Here's how the part is built. I have some questions about the finished solid (model axes, mm). A direction names the side the tool comes from. Give positions to 0.01 mm unless a question says otherwise; leave off trailing zeros. Write each loop counter-clockwise with the first axis right and the second up, starting at its lowest first coordinate (ties: lowest second). Pieces come first, ordered by that corner, then holes. Notation, with made-up numbers: M -28,84 L 22,84 A19 cw 22,106 Z; hole C 47,28.25 d1. An arc over 180 degrees is marked long. Use one line per item in the form item = value. Start each with the question number.
from build123d import *

# Parameters (mm, degrees)
F1_DEPTH = 130
F0_R     = 15
F2_DEPTH = 10
F0_R_2   = 10
F0_R_3   = 5
F3_DEPTH = 5
F4_R     = 0.8
F5_R     = 5


with BuildPart() as f1:
    # F0 (on Top) → F1 (new body)
    with BuildSketch(Plane.XY):
        with BuildLine():
            ThreePointArc((-137.9369372874, 168.1235290214), (-141.4724711934, 166.6590629273), (-142.9369372874, 163.1235290214))
            Line((-142.9369372874, 163.1235290214), (-142.9369372874, -66.8764709786))
            ThreePointArc((-142.9369372874, -66.8764709786), (-141.4724711934, -70.4120048845), (-137.9369372874, -71.8764709786))
            Line((-137.9369372874, -71.8764709786), (152.0630627126, -71.8764709786))
            ThreePointArc((152.0630627126, -71.8764709786), (155.5985966185, -70.4120048845), (157.0630627126, -66.8764709786))
            Line((157.0630627126, -66.8764709786), (157.0630627126, 163.1235290214))
            ThreePointArc((157.0630627126, 163.1235290214), (155.5985966185, 166.6590629273), (152.0630627126, 168.1235290214))
            Line((152.0630627126, 168.1235290214), (-137.9369372874, 168.1235290214))
        make_face()
        with BuildLine():
            ThreePointArc((-137.9369372874, 153.1235290214), (-135.0080050993, 160.1945968333), (-127.9369372874, 163.1235290214))
            Line((-127.9369372874, 163.1235290214), (92.0630627126, 163.1235290214))
            Line((92.0630627126, 163.1235290214), (142.0630627126, 163.1235290214))
            ThreePointArc((142.0630627126, 163.1235290214), (149.1341305244, 160.1945968333), (152.0630627126, 153.1235290214))
            Line((152.0630627126, 153.1235290214), (152.0630627126, -56.8764709786))
            ThreePointArc((152.0630627126, -56.8764709786), (149.1341305244, -63.9475387905), (142.0630627126, -66.8764709786))
            Line((142.0630627126, -66.8764709786), (92.0630627126, -66.8764709786))
            Line((92.0630627126, -66.8764709786), (-127.9369372874, -66.8764709786))
            ThreePointArc((-127.9369372874, -66.8764709786), (-135.0080050993, -63.9475387905), (-137.9369372874, -56.8764709786))
            Line((-137.9369372874, -56.8764709786), (-137.9369372874, 153.1235290214))
        make_face(mode=Mode.SUBTRACT)
    extrude(amount=F1_DEPTH)

    # F0 (on Top) → F2 (join)
    with BuildSketch(Plane.XY):
        with BuildLine():
            Line((92.0630627126, 163.1235290214), (-127.9369372874, 163.1235290214))
            ThreePointArc((-127.9369372874, 163.1235290214), (-135.0080050993, 160.1945968333), (-137.9369372874, 153.1235290214))
            Line((-137.9369372874, 153.1235290214), (-137.9369372874, -56.8764709786))
            ThreePointArc((-137.9369372874, -56.8764709786), (-135.0080050993, -63.9475387905), (-127.9369372874, -66.8764709786))
            Line((-127.9369372874, -66.8764709786), (92.0630627126, -66.8764709786))
            Line((92.0630627126, -66.8764709786), (92.0630627126, 163.1235290214))
        make_face()
        with Locations((-22.9369372874, 48.1235290214)):
            Circle(F0_R, mode=Mode.SUBTRACT)
        with BuildLine():
            Line((142.0630627126, 163.1235290214), (92.0630627126, 163.1235290214))
            Line((92.0630627126, 163.1235290214), (92.0630627126, -66.8764709786))
            Line((92.0630627126, -66.8764709786), (142.0630627126, -66.8764709786))
            ThreePointArc((142.0630627126, -66.8764709786), (149.1341305244, -63.9475387905), (152.0630627126, -56.8764709786))
            Line((152.0630627126, -56.8764709786), (152.0630627126, 153.1235290214))
            ThreePointArc((152.0630627126, 153.1235290214), (149.1341305244, 160.1945968333), (142.0630627126, 163.1235290214))
        make_face()
    extrude(amount=F2_DEPTH)



with BuildPart() as f2:
    # F0 (on Top) → F2, piece 2 (new body)
    with BuildSketch(Plane.XY):
        with Locations((-22.9369372874, 48.1235290214)):
            Circle(F0_R_2)
        with Locations((-22.9369372874, 48.1235290214)):
            Circle(F0_R_3, mode=Mode.SUBTRACT)
    extrude(amount=F2_DEPTH)


with BuildPart() as f1_1:
    add(f1.part)

    add(f2.part)  # F3 merges F2
    # F0 (on Top) → F3 (join)
    with BuildSketch(Plane.XY):
        with Locations((-22.9369372874, 48.1235290214)):
            Circle(F0_R)
        with Locations((-22.9369372874, 48.1235290214)):
            Circle(F0_R_2, mode=Mode.SUBTRACT)
    extrude(amount=F3_DEPTH)

    # F4
    f4_edges = [f1_1.edges().sort_by_distance(p)[0] for p in [
        (-32.936937, 48.123529, 10),
        (-27.936937, 48.123529, 10),
        (-37.936937, 48.123529, 10),
    ]]
    fillet(f4_edges, radius=F4_R)

    # F5
    f5_edges = [f1_1.edges().sort_by_distance(p)[0] for p in [
        (-38.736937, 48.123529, 10),
        (-135.008005, 160.194597, 10),
        (-137.936937, 48.123529, 10),
        (-135.008005, -63.947539, 10),
        (7.063063, -66.876471, 10),
        (149.134131, -63.947539, 10),
        (152.063063, 48.123529, 10),
        (149.134131, 160.194597, 10),
        (7.063063, 163.123529, 10),
    ]]
    fillet(f5_edges, radius=F5_R)


solid = f1_1.part
1) Suppose I cut it at B-B, the plane y = 89.5. List the corners of the cut face in (x, z) for me, and give its area (3 significant figures).
2) Suppose I cut it at A-A, the plane z = 106. List the corners of the cut face in (x, y) for me.
3) Thinking about a two-plate mould opening in Y: for faces 1 (the face through (5, -71.876, 64)), 2 (the face through (-24.021, 43.242, 4.536)), 3 (the face through (9, 168.124, 64)), 4 (the face through (5, 50, 0)), which applies, released by +Y, released by -Y, zero draft, split by the parting line, or undercut?
4) Suppose I cut it at C-C, the plane x = -87. List the corners of the cut face in (y, z) for me, and give its area (3 significant figures).
5) On a 3-axis mill with a long thin cutter (end or side, diameter ignored), from which of +Z, -Z, +X, -X, +Y, -Y can I reach the whole of each face in a straight line? I mean faces 5 (the face through (149.06, 160.27, 71.69)), 6 (the face through (-60, 164, 130)). Say none if no direction works.
6) Will these pins go through, and if not, where does the flat tip stop? P1, Ø12, axis at x = 80, y = 118.5, coming from the -Z side; P2, Ø2, axis at x = -69.5, y = -32, coming from the +Z side; P3, Ø6, axis at x = -22.94, y = 48.12, coming from the +Z side; P4, Ø5.5, axis at x = -24.5, y = 46, coming from the +Z side (3 decimals).
7) Please list where these lines run through material, in increasing order: line 1 (X direction, y = 143, z = 45.5); line 2 (Y direction, x = -31.5, z = 124.5); line 3 (Z direction, x = -87, y = 118).
Checks:
q1.outline = M -142.94,0 L 157.06,0 L 157.06,130 L 152.06,130 L 152.06,15 A5 cw 147.06,10 L -132.94,10 A5 cw -137.94,15 L -137.94,130 L -142.94,130 Z
q1.area = 4,210 mm^2
q2.outline = M -142.94,-66.88 A5 ccw -137.94,-71.88 L 152.06,-71.88 A5 ccw 157.06,-66.88 L 157.06,163.12 A5 ccw 152.06,168.12 L -137.94,168.12 A5 ccw -142.94,163.12 Z; hole M -137.94,-56.88 A10 ccw -127.94,-66.88 L 142.06,-66.88 A10 ccw 152.06,-56.88 L 152.06,153.12 A10 ccw 142.06,163.12 L -127.94,163.12 A10 ccw -137.94,153.12 Z
q3.face_1 = released by -Y
q3.face_2 = undercut
q3.face_3 = released by +Y
q3.face_4 = zero draft
q4.outline = M -71.88,0 L 168.12,0 L 168.12,130 L 163.12,130 L 163.12,15 A5 cw 158.12,10 L -61.88,10 A5 cw -66.88,15 L -66.88,130 L -71.88,130 Z
q4.area = 3,610 mm^2
q5.face_5 = +Z
q5.face_6 = +Z, +X, -X, +Y, -Y
q6.P1 = 0
q6.P2 = 10
q6.P3 = through
q6.P4 = 9.885
q7.line_1 = -142.94 to -137.94, 152.06 to 157.06
q7.line_2 = -71.88 to -66.88, 163.12 to 168.12
q7.line_3 = 0 to 10
